from build123d import *

# Parameters (mm, degrees)
F1_DEPTH = 60


with BuildPart() as f1:
    # F0 (on Right) → F1 (new body)
    with BuildSketch(Plane.YZ):
        with BuildLine():
            Line((-3.504068, -8.01231), (-3.504068, 6.58769))
            Line((-3.504068, 6.58769), (-5.504068, 6.58769))
            ThreePointArc((-5.504068, 6.58769), (-6.211174, 6.294796), (-6.504068, 5.58769))
            ThreePointArc((-6.504068, 5.58769), (-5.013659, -0.870279), (-7.504068, -7.01231))
            Line((-7.504068, -7.01231), (-7.504068, -8.01231))
            ThreePointArc((-7.504068, -8.01231), (-7.211174, -8.719417), (-6.504068, -9.01231))
            Line((-6.504068, -9.01231), (-3.504068, -9.01231))
            Line((-3.504068, -9.01231), (-3.504068, -8.01231))
        make_face()
        with BuildLine():
            add(Edge.make_bspline(
                [(-3.504068, 6.58769), (-3.504068, -1.169164), (-2.41404, -8.01231), (6.895932, -8.01231)],
                knots=[0, 0, 0, 0, 17.925401, 17.925401, 17.925401, 17.925401], degree=3))
            Line((-3.504068, 6.58769), (-3.504068, -8.01231))
            Line((-3.504068, -8.01231), (-3.504068, -9.01231))
            Line((-3.504068, -9.01231), (6.895932, -9.01231))
            Line((6.895932, -9.01231), (6.895932, -8.01231))
        make_face()
    extrude(amount=F1_DEPTH)


solid = f1.part
CAD build for the part. Positions are in the model's coordinates, mm. Coordinates: 2 decimals unless noted, no trailing zeros. Write item = value, one per line. Start each with the question number.
Q1. Pull direction Z, two halves, no side cores. Call faces 1 (the flat face through (30, -4, 6.588)), 2 (the flat face through (29.6, 6.896, -8.5)), 3 (the cylindrical face through (29.58, -5.007, -0.776)): pulls with the +Z half, pulls with the -Z half, needs draft (parallel to the pull), parting line crosses it, or undercut.
Q2. Flat gauge pins, fed straight in: pin 1 Ø1.5 at (x, y) = (45, 2) entering from +Z; pin 2 Ø6 at (y, z) = (1.5, 5) entering from +X; pin 3 Ø1.5 at (x, z) = (42, -5) entering from -Y; pin 4 Ø8 at (x, z) = (15.5, 5) entering from +Y. Where does each tip first touch, or does it go through?
Q3. Drill centre lines: L1, parallel to Z at x = 8.5, y = 6.25; L2, parallel to Z at x = 28.5, y = 1.5; L3, parallel to Y at x = 29.5, z = -1.5. Where is each one in solid material? Low to high.
Computed:
q1.face_1 = pulls with the +Z half
q1.face_2 = needs draft
q1.face_3 = undercut
q2.pin_1 = -6.77
q2.pin_2 = through
q2.pin_3 = -6.6
q2.pin_4 = -3.18
q3.L1 = -9.01 to -8
q3.L2 = -9.01 to -6.9
q3.L3 = -5.08 to -2.65
